```python
from build123d import *

# Parameters (mm, degrees)
F1_DEPTH = 1.5875
F3_DEPTH = 3.176
F4_R     = 1.27


with BuildPart() as f1:
    # F0 (on Front) → F1 (new body, symmetric)
    with BuildSketch(Plane.XZ):
        Polygon((12.7, 0), (0, 21.997045), (-12.7, 0), align=None)
    extrude(amount=F1_DEPTH, both=True)

    # F2 (on face) → F3 (cut, through all)
    with BuildSketch(Plane.XZ.offset(1.5875)):
        Polygon((8.300591, 2.54), (0, 16.917045), (-8.300591, 2.54), align=None)
    extrude(amount=-F3_DEPTH, mode=Mode.SUBTRACT)

    # F4
    f4_edges = [f1.edges().sort_by_distance(p)[0] for p in [
        (0, 0, 16.917045),
        (8.300591, 0, 2.54),
        (-8.300591, 0, 2.54),
    ]]
    fillet(f4_edges, radius=F4_R)


solid = f1.part
```
Here's how the part is built. I have some questions about the finished solid (model axes, mm). A direction names the side the tool comes from. Coordinates: 2 decimals unless noted, no trailing zeros. Loops run counter-clockwise (first coordinate to the right, second up) from the corner with the lowest first, then second, coordinate; pieces in that order, holes last. Notation, with made-up numbers: (-15.75, 22) - (-3.75, 22) arc R17 cw to (-3.75, 30) - close; hole circle Ø8 at (25.5, 11). An arc over 180 degrees is marked (long way). Return JSON: item names as keys, results as strings. Group by question number.
Item 1: On a 3-axis mill with a long thin cutter (end or side, diameter ignored), from which of +Z, -Z, +X, -X, +Y, -Y can I reach the whole of each face in a straight line? I mean faces 4 (the face through (0.019, 0.022, 15.647)), 5 (the face through (6.44, -0.02, 10.84)). Say none if no direction works.
Item 2: If we section it at A-A on y = -0.7: Write out the boundary of the cut face in (x, z) (3 decimals), and give its area (3 significant figures).
Item 3: We'd pull the mould along Z, two halves only. Please class faces 1 (the face through (-6.261, -0.022, 11.153)), 2 (the face through (7.21, 0.02, 3.19)), 3 (the face through (0, 0, 0)): +Z half, -Z half, draft (parallel to the pull), parting line (faces both ways), or undercut.
Item 4: If we section it at B-B on x = -4.5: Write out the boundary of the cut face in (y, z), and give its area (3 significant figures).
Item 5: I need wall thicknesses on line 1 (X direction, y = -0.1, z = 11.75); line 2 (X direction, y = 0.05, z = 5.5); line 3 (Z direction, x = -2.75, y = 0.6). Which ranges of each line are inside material? Lowest first, please. Write a range as from..to.
Item 6: Will this pin go through, and if not, where does the flat tip stop? P1, Ø1.6, axis at x = -1, y = -0.5, coming from the +Z side.
Item 7: If we section it at C-C on z = 9.25: Write out the boundary of the cut face in (x, y).
Item 8: If we section it at D-D on x = 8.75: Write out the boundary of the cut face in (y, z).
Calculated:
{
 "1": {"face 4": "+Y, -Y", "face 5": "+Z, +X, +Y, -Y"},
 "2": {"outline": "(-12.7, 0) - (12.7, 0) - (0, 21.997) - close; hole (-7.201, 4.445) arc R1.27 ccw to (-6.101, 2.54) - (6.101, 2.54) arc R1.27 ccw to (7.201, 4.445) - (1.1, 15.012) arc R1.27 ccw to (-1.1, 15.012) - close", "area": "163 mm^2"},
 "3": {"face 1": "+Z half", "face 2": "undercut", "face 3": "-Z half"},
 "4": {"outline": "(-1.59, 0) - (1.59, 0) - (1.59, 2.54) - (-1.59, 2.54) - close; (-1.59, 9.12) - (1.59, 9.12) - (1.59, 14.2) - (-1.59, 14.2) - close", "area": "24.2 mm^2"},
 "5": {"line 1": "x = -5.92..-2.98, 2.98..5.92", "line 2": "x = -9.52..-6.59, 6.59..9.52", "line 3": "z = 0..2.54, 12.15..17.23"},
 "6": {"P1": "stops at z = 21.65"},
 "7": {"outline": "(-7.36, -1.59) - (-4.43, -1.59) - (-4.43, 1.59) - (-7.36, 1.59) - close; (4.43, -1.59) - (7.36, -1.59) - (7.36, 1.59) - (4.43, 1.59) - close"},
 "8": {"outline": "(-1.59, 0) - (1.59, 0) - (1.59, 6.84) - (-1.59, 6.84) - close"}
}
